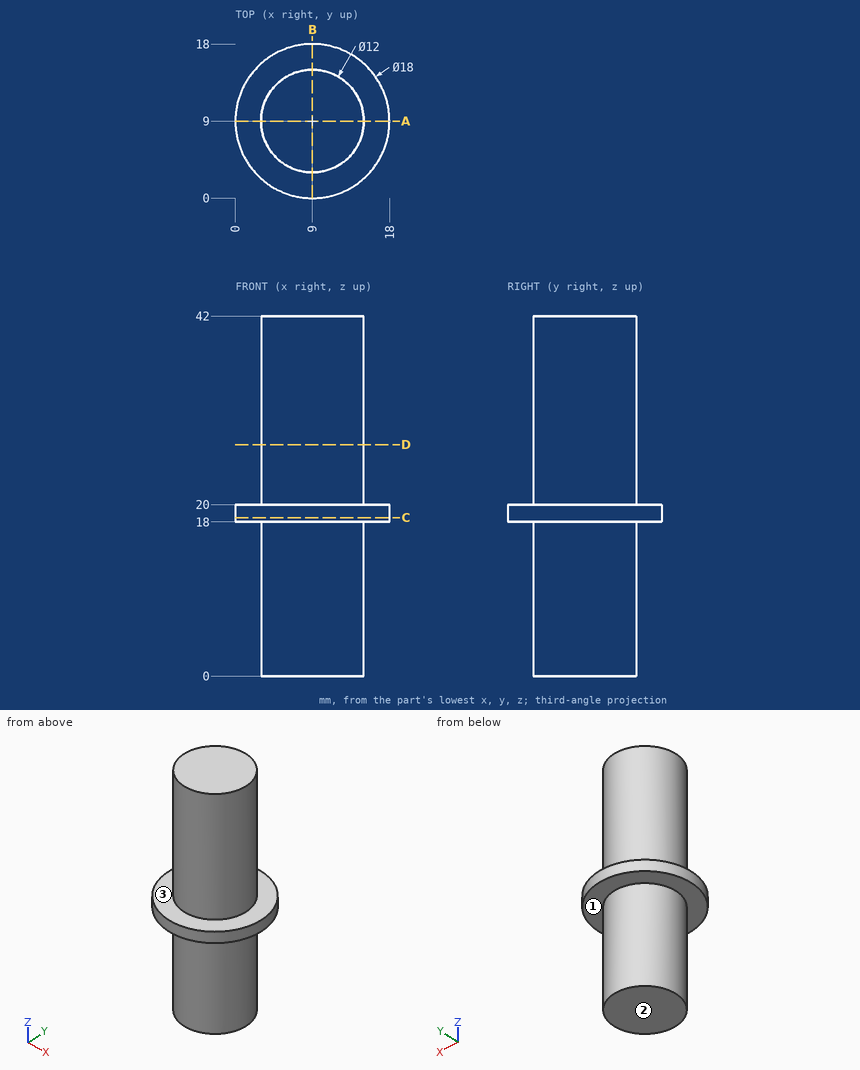
Verification items for this drawing (mm, ordinates from the low corner). A direction names the side the tool comes from. Round coordinates to 2 decimals unless told otherwise and drop trailing zeros. Order: outer loops, then holes, each group sorted by start corner. A loop starts at its lowest first (then second) coordinate and runs counter-clockwise, first axis right, second up. Notation, with made-up numbers: (46.5, 83.25) - (60.5, 83.25) arc R19 ccw to (60.5, 108.25) - close; hole circle Ø6 at (5, 0). An arc over 180 degrees is marked (long way). Use CSV: the item, a comma, the result in double quotes.
(1) Thickness scan on probe 1 along Z at (x, y) = (1.5, 7); probe 2 along X at (y, z) = (4.75, 19); probe 3 along Y at (x, z) = (7, 12). Record the ranges inside material, lowest first. Write a range as from..to.
Entries:
probe 1,"18..20"
probe 2,"1.07..16.93"
probe 3,"3.34..14.66"
(2) Section check A-A on y = 9. Record the boundary of the cut face in (x, z), and give its area (3 significant figures).
Entries:
outline,"(0, 18) - (3, 18) - (3, 0) - (15, 0) - (15, 18) - (18, 18) - (18, 20) - (15, 20) - (15, 42) - (3, 42) - (3, 20) - (0, 20) - close"
area,"516 mm^2"
(3) Section check D-D on z = 27. Record the boundary of the cut face in (x, y).
Entries:
outline,"circle Ø12 at (9, 9)"
(4) Gauge pin test, flat ends, axial feed: pin 1 Ø10 at (y, z) = (10.5, 35) entering from -X; pin 2 Ø2 at (x, y) = (15, 13) entering from +Z; pin 3 Ø4 at (x, z) = (10, 14) entering from +Y. Record the tip position at first contact, or that the pin passes through.
Entries:
pin 1,"x = 3"
pin 2,"z = 20"
pin 3,"y = 15"
(5) Section check C-C on z = 18.5. Record the boundary of the cut face in (x, y), and give its area (3 significant figures).
Entries:
outline,"circle Ø18 at (9, 9)"
area,"254 mm^2"
(6) Access from +Z, -Z, +X, -X, +Y, -Y to the whole of each face (thin tool, end or side, straight path). Record for the marked faces 1, 2 and 3.
Entries:
face 1,"-Z"
face 2,"-Z, +X, -X, +Y, -Y"
face 3,"+Z"
